Verification items for the finished model (mm, model axes). Coordinates: 2 decimals unless noted, no trailing zeros. Order: outer loops, then holes, each group sorted by start corner. A loop starts at its lowest first (then second) coordinate and runs counter-clockwise, first axis right, second up. Notation, with made-up numbers: (80, -19) -> (101, -19) arc R22 ccw to (101, 0) -> close; hole circle Ø7 at (-8, 19.25). An arc over 180 degrees is marked (long way). Write item = value, one per line. Start each with the question number.
1. Cross-section at A-A on x = 1.5. Record the cut outline in (y, z), plus the area to 3 significant figures.
2. Go/stop test with a flat-tipped pin: P1, Ø2, axis at x = 9.5, z = 1.5, coming from the +Y side. Record where the tip stops, or that it passes through.
3. Thickness scan on line 1 along X through (y, z) = (-113, 3.5); line 2 along Z through (x, y) = (10.5, -40.5). Record the ranges inside material, lowest first. Write a range as from..to.
4. Cross-section at B-B on y = -57.5. Record the cut outline in (x, z).
5. Cross-section at C-C on z = 9.5. Record the cut outline in (x, y), plus the area to 3 significant figures.
6. Cross-section at D-D on x = 10.25. Record the cut outline in (y, z), plus the area to 3 significant figures.
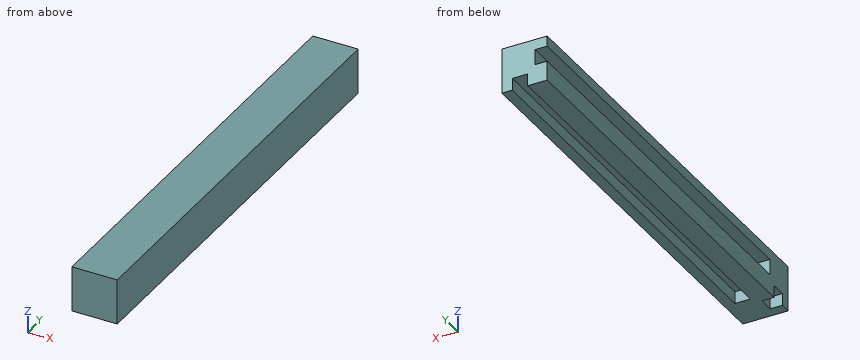
from build123d import *

# Parameters (mm, degrees)
F1_DEPTH      = 138
F2_W          = 15
F2_H          = 15
F3_DEPTH      = 7
F3_DEPTH_BACK = 4
F4_W          = 4
F4_H          = 5
F5_DEPTH      = 4


with BuildPart() as f1:
    # F0 (on Front) → F1 (new body)
    with BuildSketch(Plane.XZ):
        Polygon((0, 6.45), (0, 0), (6.45, 0), (6.45, 4), (11.55, 4), (11.55, 0), (15, 0), (15, 15), (0, 15), (0, 11.55), (4, 11.55), (4, 6.45), align=None)
    extrude(amount=F1_DEPTH)

    # F2 (on face) → F3 (join, two sides)
    with BuildSketch(Plane.XZ.offset(138)) as f3_sk:
        with Locations((7.5, 7.5)):
            Rectangle(F2_W, F2_H)
    extrude(amount=F3_DEPTH)
    extrude(f3_sk.sketch, amount=-F3_DEPTH_BACK)

    # F4 (on face) → F5 (cut)
    with BuildSketch(Plane(origin=(0, 0, 0), x_dir=(1, 0, 0), z_dir=(0, 0, -1))):
        with Locations((2, 139)):
            Rectangle(F4_W, F4_H)
    extrude(amount=-F5_DEPTH, mode=Mode.SUBTRACT)


solid = f1.part
Worked out:
q1.outline = (-145, 0) -> (-141.5, 0) -> (-141.5, 4) -> (-136.5, 4) -> (-136.5, 0) -> (0, 0) -> (0, 6.45) -> (-134, 6.45) -> (-134, 11.55) -> (0, 11.55) -> (0, 15) -> (-145, 15) -> close
q1.area = 1,470 mm²
q2.P1 = -134
q3.line_1 = 0..6.45, 11.55..15
q3.line_2 = 4..15
q4.outline = (0, 0) -> (6.45, 0) -> (6.45, 4) -> (11.55, 4) -> (11.55, 0) -> (15, 0) -> (15, 15) -> (0, 15) -> (0, 11.55) -> (4, 11.55) -> (4, 6.45) -> (0, 6.45) -> close
q5.outline = (0, -145) -> (15, -145) -> (15, 0) -> (4, 0) -> (4, -134) -> (0, -134) -> close
q5.area = 1,640 mm²
q6.outline = (-145, 0) -> (-134, 0) -> (-134, 4) -> (0, 4) -> (0, 15) -> (-145, 15) -> close
q6.area = 1,640 mm²
